```python
from build123d import *

# Parameters (mm, degrees)
F0_W     = 127
F0_H     = 49.53
F1_DEPTH = 19.05
F2_W     = 25.4
F2_H     = 49.53
F3_DEPTH = 10.16
F4_DEPTH = 10.16
F2_R     = 3.175
F5_DEPTH = 9.525
F6_SIZE  = 6.35
F7_R     = 3.175


with BuildPart() as f1:
    # F0 (on Top) → F1 (new body)
    with BuildSketch(Plane.XY):
        Rectangle(F0_W, F0_H)
    extrude(amount=F1_DEPTH)

    # F2 (on face) → F3 (cut)
    with BuildSketch(Plane.XY.offset(19.05)):
        with Locations((-38.1, 0)):
            Rectangle(F2_W, F2_H)
    extrude(amount=-F3_DEPTH, mode=Mode.SUBTRACT)

    # F2 (on face) → F4 (cut)
    with BuildSketch(Plane.XY.offset(19.05)):
        with Locations((38.6475931525, 0)):
            Rectangle(F2_W, F2_H)
    extrude(amount=-F4_DEPTH, mode=Mode.SUBTRACT)

    # F2 (on face) → F5 (cut)
    with BuildSketch(Plane.XY.offset(19.05)):
        with Locations((-6.35, -12.3330028728)):
            Circle(F2_R)
        with Locations((-12.7, 0)):
            Circle(F2_R)
        with Locations((-6.35, 12.3330028728)):
            Circle(F2_R)
        with Locations((12.7, 13.2446838543)):
            Circle(F2_R)
        with Locations((15.875, 0)):
            Circle(F2_R)
        with Locations((12.7, -13.2446838543)):
            Circle(F2_R)
    extrude(amount=-F5_DEPTH, mode=Mode.SUBTRACT)

    # F6
    f6_edges = [f1.edges().sort_by_distance(p)[0] for p in [
        (63.5, -24.765, 9.525),
        (63.5, 24.765, 9.525),
        (-63.5, -24.765, 9.525),
        (-63.5, 24.765, 9.525),
    ]]
    chamfer(f6_edges, length=F6_SIZE)

    # F7
    f7_edges = [f1.edges().sort_by_distance(p)[0] for p in [
        (-57.15, -24.765, 9.525),
        (57.15, -24.765, 9.525),
        (63.5, -18.415, 9.525),
        (63.5, 18.415, 9.525),
        (-63.5, -18.415, 9.525),
        (57.15, 24.765, 9.525),
        (-57.15, 24.765, 9.525),
        (-63.5, 18.415, 9.525),
    ]]
    fillet(f7_edges, radius=F7_R)


solid = f1.part
```
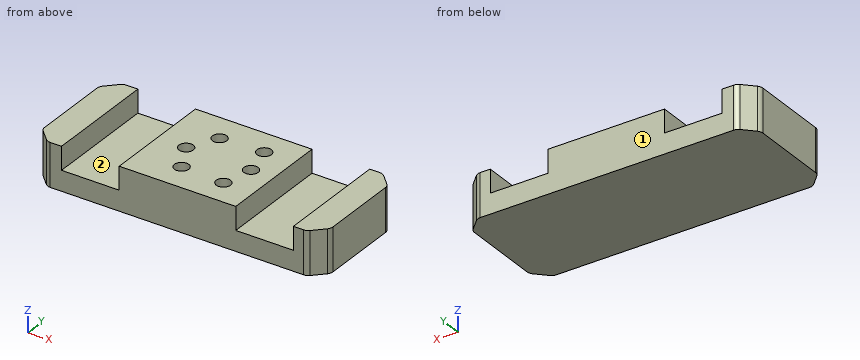
Could you check a few things on this model? Use its own coordinates, in mm. Face numbers are marked on the shaded views. A direction names the side the tool comes from. Round coordinates to 2 decimals unless told otherwise and drop trailing zeros. Loops run counter-clockwise (first coordinate to the right, second up) from the corner with the lowest first, then second, coordinate; pieces in that order, holes last. Notation, with made-up numbers: (22, 34.25) - (29, 34.25) arc R18 cw to (29, 40.25) - close; hole circle Ø4 at (12, -19.75). An arc over 180 degrees is marked (long way). Answer in a Markdown table with one row per item. Add a question column.
(1) If we section it at C-C (y = 0): Please give me the cut outline in (x, z) (3 decimals), plus the area to 3 significant figures.
(2) I need wall thicknesses on line 1 along X through (y, z) = (5, 10); line 2 along X through (y, z) = (-13.5, 10); line 3 along X through (y, z) = (22, 15.25) (3 decimals). Which ranges of each line are inside material? Lowest first, please.
(3) If we section it at D-D (y = 5.5): Please give me the cut outline in (x, z), plus the area to 3 significant figures.
(4) I'm going to push flat-ended pins straight in: pin 1 (7.5 mm diameter, centred on x = -38, y = -5, fed in from +Z); pin 2 (3 mm diameter, centred on x = -13, y = 1.5, fed in from +Z) (3 decimals); pin 3 (1 mm diameter, centred on y = 18.5, z = 13, fed in from -X). Where does each tip first touch, or does it pass through?
(5) If we section it at B-B (x = -6.35): Please give me the cut outline in (y, z) (3 decimals).
(6) For the marked faces 1 and 2, which set-ups out of +Z, -Z, +X, -X, +Y, -Y let a thin tool reach every point of the face, with its end or its side?
(7) If we section it at A-A (z = 17): State how many separate pieces and enclosed holes the cut face has, plus the area to 3 significant figures.
Model answer:
| question | item | result |
|---|---|---|
| 1 | outline | (-63.5, 0) - (63.5, 0) - (63.5, 19.05) - (51.348, 19.05) - (51.348, 8.89) - (25.948, 8.89) - (25.948, 19.05) - (19.05, 19.05) - (19.05, 9.525) - (12.7, 9.525) - (12.7, 19.05) - (-9.525, 19.05) - (-9.525, 9.525) - (-15.875, 9.525) - (-15.875, 19.05) - (-25.4, 19.05) - (-25.4, 8.89) - (-50.8, 8.89) - (-50.8, 19.05) - (-63.5, 19.05) - close |
| 1 | area | 1,780 mm² |
| 2 | line 1 | x = -63.5 to -50.8, -25.4 to 25.95, 51.35 to 63.5 |
| 2 | line 2 | x = -63.5 to -50.8, -25.4 to -9.3, -3.4 to 9.54, 15.86 to 25.95, 51.35 to 63.5 |
| 2 | line 3 | x = -59.915 to -50.8, -25.4 to 25.948, 51.348 to 59.915 |
| 3 | outline | (-63.5, 0) - (63.5, 0) - (63.5, 19.05) - (51.35, 19.05) - (51.35, 8.89) - (25.95, 8.89) - (25.95, 19.05) - (-25.4, 19.05) - (-25.4, 8.89) - (-50.8, 8.89) - (-50.8, 19.05) - (-63.5, 19.05) - close |
| 3 | area | 1,900 mm² |
| 4 | pin 1 | stops at z = 8.89 |
| 4 | pin 2 | stops at z = 9.525 |
| 4 | pin 3 | stops at x = -63.37 |
| 5 | outline | (-24.765, 0) - (24.765, 0) - (24.765, 19.05) - (15.508, 19.05) - (15.508, 9.525) - (9.158, 9.525) - (9.158, 19.05) - (-9.158, 19.05) - (-9.158, 9.525) - (-15.508, 9.525) - (-15.508, 19.05) - (-24.765, 19.05) - close |
| 6 | face 1 | +Z, -Z, +X, -X, +Y |
| 6 | face 2 | +Z, +Y, -Y |
| 7 | separate pieces | 3 |
| 7 | enclosed holes | 6 |
| 7 | area | 3,500 mm² |
